```python
from build123d import *

# Parameters (mm, degrees)
CROQUIS1_R              = 7.575
SALIENTE_EXTRUIR1_DEPTH = 25.5
BOSS_EXTRUDE1_DEPTH     = 25.5
SKETCH7_R               = 11
CUT_EXTRUDE1_DEPTH      = 3.5
SKETCH9_R               = 5.25
CUT_EXTRUDE3_DEPTH      = 22
REDONDEO1_R             = 10
FILLET1_R               = 5
SKETCH8_R               = 4.75
CUT_EXTRUDE2_DEPTH      = 88.312260382
SKETCH11_R              = 2.05
CUT_EXTRUDE4_DEPTH      = 10


with BuildPart() as part:
    # Croquis1 → Saliente-Extruir1 (new body)
    with BuildSketch(Plane.XY):
        Polygon((79.406412185, 15.36568027), (79.406412185, 34.441404803), (102.206412031, 34.441404803), (102.206412031, 13.841404803), (91.906412031, 1.820896426), (36.506412031, 1.820896426), (26.206412031, 13.841404803), (26.206412031, 34.441404803), (49.006411878, 34.441404803), (49.006411878, 15.36568027), (64.10641184, 6.647691683), (64.206412031, 6.589956548), (64.306412223, 6.647691683), align=None)
        with Locations((91.906412031, 24.141404803)):
            Circle(CROQUIS1_R, mode=Mode.SUBTRACT)
        with Locations(Location((36.506412031, 24.141404803, 0), (0, 0, 180))):
            Circle(CROQUIS1_R, mode=Mode.SUBTRACT)
    extrude(amount=-SALIENTE_EXTRUIR1_DEPTH)

    # Sketch4 → Boss-Extrude1 (add)
    with BuildSketch(Plane.XY):
        Polygon((64.206412031, 6.589956548), (79.406412185, 15.36568027), (79.406412185, 64.36568027), (71.206412031, 64.36568027), (71.206412031, 38.80809142), (57.206412031, 38.80809142), (57.206412031, 64.36568027), (49.006411878, 64.36568027), (49.006411878, 15.36568027), align=None)
    extrude(amount=-BOSS_EXTRUDE1_DEPTH)

    # Sketch7 → Cut-Extrude1 (cut)
    with BuildSketch(Plane.XY):
        with Locations((64.206412031, 24.141404803)):
            Circle(SKETCH7_R)
    extrude(amount=-CUT_EXTRUDE1_DEPTH, mode=Mode.SUBTRACT)

    # Sketch9 → Cut-Extrude3 (cut)
    with BuildSketch(Plane.XY.offset(-3.5)):
        with Locations((64.206412031, 24.141404803)):
            Circle(SKETCH9_R)
    extrude(amount=-CUT_EXTRUDE3_DEPTH, mode=Mode.SUBTRACT)

    # Redondeo1
    redondeo1_edges = [part.edges().sort_by_distance(p)[0] for p in [
        (102.206412031, 34.441404803, -12.75),
        (26.206412031, 34.441404803, -12.75),
    ]]
    fillet(redondeo1_edges, radius=REDONDEO1_R)

    # Fillet1
    fillet1_edges = [part.edges().sort_by_distance(p)[0] for p in [
        (102.206412031, 13.841404803, -12.75),
        (91.906412031, 1.820896426, -12.75),
        (36.506412031, 1.820896426, -12.75),
        (26.206412031, 13.841404803, -12.75),
    ]]
    fillet(fillet1_edges, radius=FILLET1_R)

    # Sketch8 → Cut-Extrude2 (cut, through all)
    with BuildSketch(Plane(origin=(79.406412185, 0, 0), x_dir=(0, 0, -1), z_dir=(1, 0, 0))):
        with Locations((12.75, 49.403542537)):
            Circle(SKETCH8_R)
    extrude(amount=-CUT_EXTRUDE2_DEPTH, mode=Mode.SUBTRACT)

    # Sketch11 → Cut-Extrude4 (cut)
    with BuildSketch(Plane.XY.offset(-3.5)):
        with Locations((72.206412031, 24.141404803)):
            Circle(SKETCH11_R)
        with Locations((64.206412031, 32.141404803)):
            Circle(SKETCH11_R)
        with Locations((56.206412031, 24.141404803)):
            Circle(SKETCH11_R)
        with Locations((64.206412031, 16.141404803)):
            Circle(SKETCH11_R)
    extrude(amount=-CUT_EXTRUDE4_DEPTH, mode=Mode.SUBTRACT)


solid = part.part
```
Design review of the part built by this model. Coordinates are the model's own, in mm. A direction names the side the tool comes from. Give positions to 0.01 mm unless a question says otherwise; leave off trailing zeros. Order: outer loops, then holes, each group sorted by start corner. A loop starts at its lowest first (then second) coordinate and runs counter-clockwise, first axis right, second up. Notation, with made-up numbers: (4.5, -38) - (53.5, -38) arc R12 cw to (53.5, -33) - close; hole circle Ø9 at (-26.5, 79). An arc over 180 degrees is marked (long way). Use a Markdown table: item, result. Add a question column.
(1) Add section A-A on y = 43.5. Give the boundary of the cut face in (x, z), then the cut area to 3 significant figures.
(2) Wall thickness on probe 1 along X at (y, z) = (41, -12); probe 2 along X at (y, z) = (19.5, -20.25); probe 3 along X at (y, z) = (20.5, -12.75): over which ranges is each line inside the solid? List them lowest first. Write a range as [from, to].
(3) Machinability: for faces 5 (the face through (64, 38.808, -13)), 6 (the face through (75.364, 44.766, -11.72)), 7 (the face through (55, 27, -25.5)), 8 (the face through (79.406, 49, -18)), 9 (the face through (62.7, 33.53, -8.43)), which of the approach directions +Z, -Z, +X, -X, +Y, -Y give a long, thin tool a straight path to every point of the face, cutting with its end or side? Answer none if there is none.
(4) Add section D-D on y = 27.5. Give the boundary of the cut face in (x, z).
(5) Clearance check with flat-ended pins moving along their axes: P1, Ø13, axis at y = 54, z = -10, coming from the +X side; P2, Ø10, axis at x = 85, z = -9.5, coming from the +Y side; P3, Ø4, axis at y = 35.5, z = -18, coming from the +X side; P4, Ø9.5, axis at x = 64.21, y = 24.14, coming from the +Z side. State where each tip first meets the part, or that it passes through.
(6) Add section C-C on z = -14.5. Give the number of separate pieces and of enclosed holes in the cut face, then the cut area to 3 significant figures.
(7) Add section B-B on x = 96. Give the boundary of the cut face in (y, z).
(8) Mouldability with a two-part tool opening along X and no side actions: class faces 1 (the face through (26.206, 20, -13)), 2 (the face through (56, 24, -13.5)), 3 (the face through (57.206, 54, -10)), 4 (the face through (65, 1.821, -13)) as +X half, -X half, draft (parallel to the pull), parting line (faces both ways), or undercut.
Report:
| question | item | result |
|---|---|---|
| 1 | outline | (49.01, -25.5) - (57.21, -25.5) - (57.21, 0) - (49.01, 0) - close; (71.21, -25.5) - (79.41, -25.5) - (79.41, 0) - (71.21, 0) - close |
| 1 | area | 418 mm² |
| 2 | probe 1 | x = [49.01, 57.21], [71.21, 79.41] |
| 2 | probe 2 | x = [26.21, 30.52], [42.49, 61.75], [66.66, 85.92], [97.89, 102.21] |
| 2 | probe 3 | x = [26.21, 29.86], [43.15, 60.42], [67.99, 85.26], [98.55, 102.21] |
| 3 | face 5 | +Z, -Z, +Y |
| 3 | face 6 | +X, -X |
| 3 | face 7 | -Z, +X, -X, +Y, -Y |
| 3 | face 8 | +Z, -Z, +X, +Y |
| 3 | face 9 | +Z |
| 4 | outline | (26.69, -25.5) - (29.72, -25.5) - (29.72, 0) - (26.69, 0) - close; (43.3, -25.5) - (60.17, -25.5) - (60.17, -3.5) - (53.73, -3.5) - (53.73, 0) - (43.3, 0) - close; (68.24, -25.5) - (85.12, -25.5) - (85.12, 0) - (74.68, 0) - (74.68, -3.5) - (68.24, -3.5) - close; (98.7, -25.5) - (101.73, -25.5) - (101.73, 0) - (98.7, 0) - close |
| 5 | P1 | stops at x = 79.41 |
| 5 | P2 | stops at y = 34.44 |
| 5 | P3 | stops at x = 96.44 |
| 5 | P4 | passes through |
| 6 | separate pieces | 3 |
| 6 | enclosed holes | 3 |
| 6 | area | 2,270 mm² |
| 7 | outline | (6.6, -25.5) - (17.77, -25.5) - (17.77, 0) - (6.6, 0) - close; (30.52, -25.5) - (33.69, -25.5) - (33.69, 0) - (30.52, 0) - close |
| 8 | face 1 | -X half |
| 8 | face 2 | undercut |
| 8 | face 3 | undercut |
| 8 | face 4 | draft |
